Job drawing, mm, ordinate dimensions from the low corner. One solid piece. A direction names the side the tool comes from. Round coordinates to 2 decimals unless told otherwise and drop trailing zeros. Write each loop counter-clockwise with the first axis right and the second up, starting at its lowest first coordinate (ties: lowest second). Pieces come first, ordered by that corner, then holes. Notation, with made-up numbers: M 27,88 L 78,88 A25 ccw 78,100 Z; hole C 6,-26 d6. An arc over 180 degrees is marked long. Answer as a JSON object with one key per item and string values. Group by question number.
1. Two-plate mould, pull along Y, no slides. Class the marked faces 1, 2 and 3: +Y half, -Y half, draft (parallel to the pull), parting line (faces both ways), or undercut.
2. Band-saw the part on A-A, the plane y = 6.25. Write the cut outline in (x, z).
3. Band-saw the part on B-B, the plane x = 9. Write the cut outline in (y, z), plus the area to 3 significant figures.
4. Which spindle directions (+Z, -Z, +X, -X, +Y, -Y) get a long thin tool onto all of the face, cutting with end or side? Do the marked faces 4 and 5. Say none if no direction does.
5. Band-saw the part on C-C, the plane z = 2.55. Write the cut outline in (x, y) (3 decimals).
6. Band-saw the part on D-D, the plane x = 3. Write the cut outline in (y, z), plus the area to 3 significant figures.
7. Drill centre lines: line 1 (Y direction, x = 6.75, z = 3.7); line 2 (Z direction, x = 4.75, y = 1.75); line 3 (X direction, y = 7.25, z = 0.3). Where is each one in solid material? Low to high. Write a range as from..to.
8. Drop flat-ended pins along their axis: pin 1 (1.5 mm diameter, centred on x = 10.5, y = 3, fed in from -Z); pin 2 (1.5 mm diameter, centred on y = 3.5, z = 2, fed in from -X). Give the stop position or say it passes through.
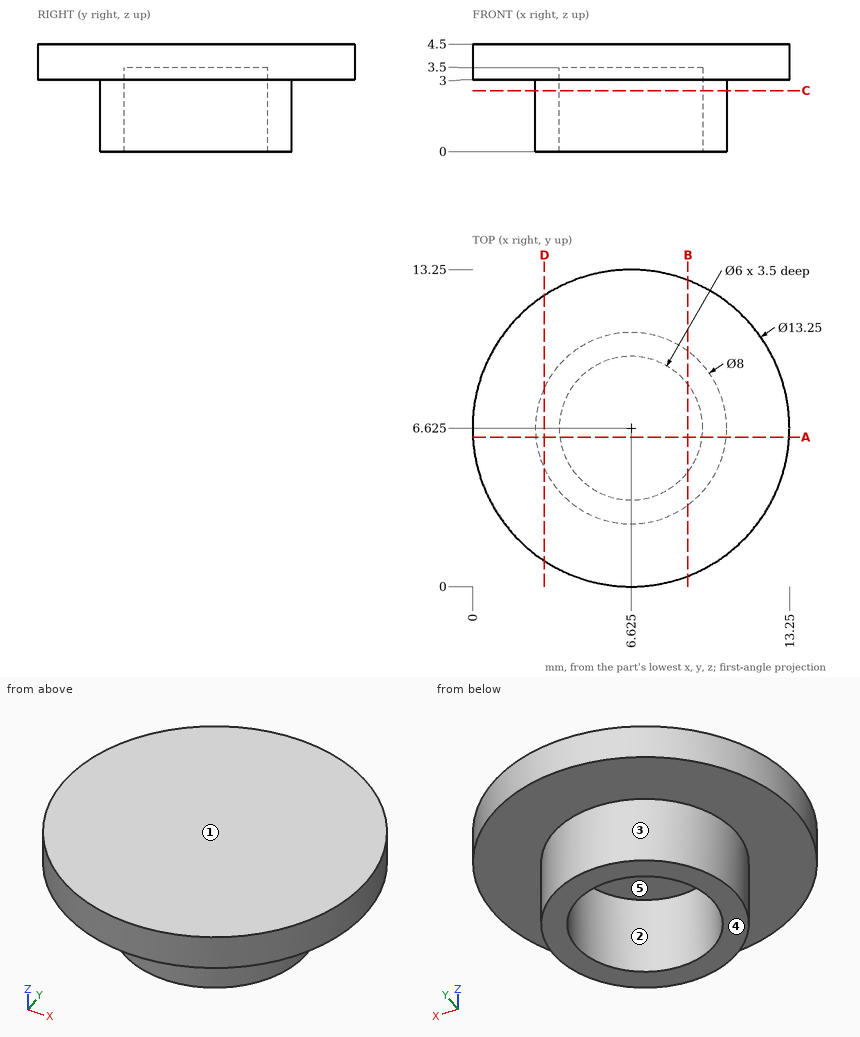
Worked answers:
{
 "1": {"face 1": "draft", "face 2": "undercut", "face 3": "parting line"},
 "2": {"outline": "M 0.01,3 L 2.64,3 L 2.64,0 L 3.65,0 L 3.65,3.5 L 9.6,3.5 L 9.6,0 L 10.61,0 L 10.61,3 L 13.24,3 L 13.24,4.5 L 0.01,4.5 Z"},
 "3": {"outline": "M 0.44,3 L 3.41,3 L 3.41,0 L 4.79,0 L 4.79,3.5 L 8.46,3.5 L 8.46,0 L 9.84,0 L 9.84,3 L 12.81,3 L 12.81,4.5 L 0.44,4.5 Z", "area": "25.0 mm^2"},
 "4": {"face 4": "-Z, +X, -X, +Y, -Y", "face 5": "-Z"},
 "5": {"outline": "C 6.625,6.625 d8; hole C 6.625,6.625 d6"},
 "6": {"outline": "M 1.08,3 L 4.93,3 L 4.93,0 L 8.32,0 L 8.32,3 L 12.17,3 L 12.17,4.5 L 1.08,4.5 Z", "area": "26.8 mm^2"},
 "7": {"line 1": "y = 0..13.25", "line 2": "z = 3..4.5", "line 3": "x = 2.67..3.69, 9.56..10.58"},
 "8": {"pin 1": "stops at z = 3", "pin 2": "stops at x = 3.41"}
}
